Check sheet for the modelled part. Datum: model origin and axes. Units: mm. A direction names the side the tool comes from. Give positions to 0.01 mm unless a question says otherwise; leave off trailing zeros. Loops run counter-clockwise (first coordinate to the right, second up) from the corner with the lowest first, then second, coordinate; pieces in that order, holes last.
Autodesk Inventor part; units mm, degrees
ref_plane "YZ Plane" through (0, 0, 0) normal (1, 0, 0) x (0, 1, 0)
ref_plane "XZ Plane" through (0, 0, 0) normal (0, 1, 0) x (-1, 0, 0)
ref_plane "XY Plane" through (0, 0, 0) normal (0, 0, 1) x (1, 0, 0)
sketch "Esquisse1" plane through (0, 0, 0) normal (0, 0, 1) x (1, 0, 0)
  line L0 (0, 0) -> (18.3, 0)
  line L1 (18.3, 0) -> (18.3, 2.2)
  line L2 (18.3, 2.2) -> (-2.2, 2.2)
  line L3 (-2.2, 2.2) -> (-2.2, -18.3)
  line L4 (-2.2, -18.3) -> (0, -18.3)
  line L5 (0, -18.3) -> (0, 0)
  dimension "Epaisseur_cornière" = 2.2
  dimension "Largueur" = 20.5
extrude "Embase" add sketch "Esquisse1" along normal mid plane 401.4
sketch "Esquisse2" plane through (0, 0, 0) normal (0, 1, 0) x (-1, 0, 0)
  line L0 (2.2, 200.7) -> (-18.3, 180.2)
  line L1 (-18.3, 180.2) -> (-18.3, 200.7)
  line L2 (-18.3, 200.7) -> (2.2, 200.7)
  line L3 (-18.3, 200.7) -> (2.2, 200.7) construction
  line L4 (2.2, -200.7) -> (2.2, 200.7) construction
  line L5 (-18.3, -200.7) -> (-18.3, 200.7) construction
  point P0 (0, 0)
  dimension "d4" = 45
extrude "Découpe à 45" cut sketch "Esquisse2" along normal through all both and the other way through all
mirror "Symétrie découpe" about plane through (0, 0, 0) normal (0, 0, 1) of "Découpe à 45"
properties part number "Profilé superieur face" material "Aluminium 6061"
(1) Section check A-A on y = -4. Record the boundary of the cut face in (x, z).
(2) Material ranges on line 1 (Y direction, x = 9, z = -97); line 2 (X direction, y = -2.75, z = -150.5), recorded low to high.
(3) Access from +Z, -Z, +X, -X, +Y, -Y to the whole of each face (thin tool, end or side, straight path). Record for faces 1 (the face through (0, -9, -3)), 2 (the face through (3.4, 0.3, 195.1)).
(4) Section check B-B on z = -41.5. Record the boundary of the cut face in (x, y).
(5) Gauge pin test, flat ends, axial feed: pin 1 Ø9 at (y, z) = (-13.5, 70) entering from +X; pin 2 Ø12 at (x, z) = (8, -15.5) entering from -Y; pin 3 Ø8 at (y, z) = (-1.5, 136.5) entering from +X. Record the tip position at first contact, or that the pin passes through.
(6) Section check C-C on x = 12. Record the boundary of the cut face in (y, z).
Computed values:
1. outline: (-2.2, -200.7) - (0, -198.5) - (0, 198.5) - (-2.2, 200.7) - close
2. line 1: y = 0 to 2.2
2. line 2: x = -2.2 to 0
3. face 1: +Z, -Z, +X, -Y
3. face 2: +Z, +X, +Y, -Y
4. outline: (-2.2, -18.3) - (0, -18.3) - (0, 0) - (18.3, 0) - (18.3, 2.2) - (-2.2, 2.2) - close
5. pin 1: stops at x = 0
5. pin 2: stops at y = 0
5. pin 3: stops at x = 18.3
6. outline: (0, -186.5) - (2.2, -186.5) - (2.2, 186.5) - (0, 186.5) - close
